```python
from build123d import *

# Parameters (mm, degrees)
SKETCH2_W                      = 99
SKETCH2_H                      = 69
SKETCH2_R                      = 25
BOSS_EXTRUDE1_DEPTH            = 10
BOSS_EXTRUDE2_DEPTH            = 120
CBORE_FOR_M5_SHCS1_D           = 5.5
CBORE_FOR_M5_SHCS1_CBORE_D     = 8
CBORE_FOR_M5_SHCS1_CBORE_DEPTH = 7
M5_CLEARANCE_HOLE1_D           = 5.5
M5_CLEARANCE_HOLE2_D           = 5.5
M5_CLEARANCE_HOLE2_DEPTH       = 10
SKETCH11_W                     = 10
SKETCH11_H                     = 120
BOSS_EXTRUDE3_DEPTH            = 13.5
FILLET1_R                      = 20
FILLET2_R                      = 10


with BuildPart() as part:
    # Sketch2 → Boss-Extrude1 (new body)
    with BuildSketch(Plane(origin=(0, 0, 0), x_dir=(1, 0, 0), z_dir=(0, 1, 0))):
        with Locations((0, -4.5)):
            Rectangle(SKETCH2_W, SKETCH2_H)
        with Locations(Location((0, 0, 0), (0, 0, 270))):
            Circle(SKETCH2_R, mode=Mode.SUBTRACT)
    extrude(amount=BOSS_EXTRUDE1_DEPTH)

    # Sketch3 → Boss-Extrude2 (add)
    with BuildSketch(Plane.XZ):
        Polygon((-49.5, -30), (-49.5, 39), (49.5, 39), (49.5, -30), (39.5, -30), (39.5, 29), (-39.5, 29), (-39.5, -30), align=None)
    extrude(amount=BOSS_EXTRUDE2_DEPTH)

    # CBORE for M5 SHCS1 (through all)
    with Locations(Plane(origin=(0, 10, 0), x_dir=(1, 0, 0), z_dir=(0, 1, 0))):
        with Locations((24.748737342, 24.748737342), (-24.748737342, 24.748737342), (24.748737342, -24.748737342), (-24.748737342, -24.748737342)):
            CounterBoreHole(CBORE_FOR_M5_SHCS1_D / 2, CBORE_FOR_M5_SHCS1_CBORE_D / 2, CBORE_FOR_M5_SHCS1_CBORE_DEPTH)

    # M5 Clearance Hole1 (through all)
    with Locations(Plane.XY.offset(39)):
        with Locations((-12.5, -60), (12.5, -110), (-12.5, -110), (12.5, -60)):
            Hole(M5_CLEARANCE_HOLE1_D / 2)

    # M5 Clearance Hole2
    with Locations(Plane(origin=(49.5, 0, 0), x_dir=(0, 0, -1), z_dir=(1, 0, 0))):
        with Locations((0, -60), (0, -110)):
            Hole(M5_CLEARANCE_HOLE2_D / 2, depth=M5_CLEARANCE_HOLE2_DEPTH)

    # Sketch11 → Boss-Extrude3 (add)
    with BuildSketch(Plane(origin=(-39.5, 0, 0), x_dir=(0, 0, -1), z_dir=(1, 0, 0))):
        with Locations((25, -60)):
            Rectangle(SKETCH11_W, SKETCH11_H)
    extrude(amount=BOSS_EXTRUDE3_DEPTH)

    # Fillet1
    fillet1_edges = [part.edges().sort_by_distance(p)[0] for p in [
        (49.5, -55, 39),
        (-49.5, -55, 39),
    ]]
    fillet(fillet1_edges, radius=FILLET1_R)

    # Fillet2
    # the kernel refuses this fillet: 10 mm, written as the material it adds along each edge
    with BuildSketch(Plane(origin=(39.5, 0, -30), x_dir=(0, -1, 0), z_dir=(0, 0, 1))) as fillet2_piece_1:
        with BuildLine():
            CenterArc((FILLET2_R, -FILLET2_R), FILLET2_R, 90, 90)
            Line((0, -FILLET2_R), (0, 0))
            Line((0, 0), (FILLET2_R, 0))
        make_face()
    extrude(amount=59)
    with BuildSketch(Plane(origin=(-39.5, 0, 29), x_dir=(1, 0, 0), z_dir=(0, 0, -1))) as fillet2_piece_2:
        with BuildLine():
            CenterArc((FILLET2_R, FILLET2_R), FILLET2_R, 180, 90)
            Line((0, FILLET2_R), (0, 0))
            Line((0, 0), (FILLET2_R, 0))
        make_face()
    extrude(amount=49)
    with BuildSketch(Plane(origin=(-39.5, 0, 29), x_dir=(0, 0, -1), z_dir=(0, -1, 0))) as fillet2_piece_3:
        with BuildLine():
            CenterArc((FILLET2_R, FILLET2_R), FILLET2_R, 180, 90)
            Line((0, FILLET2_R), (0, 0))
            Line((0, 0), (FILLET2_R, 0))
        make_face()
    extrude(amount=120)
    with BuildSketch(Plane(origin=(39.5, 0, 29), x_dir=(0, 0, -1), z_dir=(0, -1, 0)), Plane(origin=(-39.5, -120, -20), x_dir=(1, 0, 0), z_dir=(0, 1, 0))) as fillet2_piece_4:
        with BuildLine():
            CenterArc((FILLET2_R, -FILLET2_R), FILLET2_R, 90, 90)
            Line((0, -FILLET2_R), (0, 0))
            Line((0, 0), (FILLET2_R, 0))
        make_face()
    extrude(amount=120)
    with BuildSketch(Plane(origin=(-26, 0, -2.197582327), x_dir=(1, 0, 0), z_dir=(0, 0, -1))) as fillet2_piece_5_section:
        with BuildLine():
            CenterArc((FILLET2_R, FILLET2_R), FILLET2_R, 180, 90)
            Line((0, FILLET2_R), (0, 0))
            Line((0, 0), (FILLET2_R, 0))
        make_face()
    fillet2_piece_5 = extrude(amount=27.802417673, mode=Mode.PRIVATE)
    fillet2_piece_5 = split(fillet2_piece_5, bisect_by=Plane(origin=(-18.601224516, -0.292097945, -20), z_dir=(0, 0, -1)), keep=Keep.TOP, mode=Mode.PRIVATE)
    fillet2_piece_5 = fillet2_piece_5 - Plane(origin=(-24.748737342, -0.292097945, -24.748737342), x_dir=(-1, 0, 0), z_dir=(0, -1, 0)) * Cylinder(2.75, 96, mode=Mode.PRIVATE)
    add(fillet2_piece_5)


solid = part.part
```
Input: part model. Units: mm. Frame: model coordinates. A direction names the side the tool comes from. Coordinates: 2 decimals unless noted, no trailing zeros. Order: outer loops, then holes, each group sorted by start corner. A loop starts at its lowest first (then second) coordinate and runs counter-clockwise, first axis right, second up. Notation, with made-up numbers: (-13.5, 35) - (12.5, 35) arc R16 cw to (12.5, 64) - close; hole circle Ø9 at (44.25, 65.5). An arc over 180 degrees is marked (long way). Put each result on its own line as item: value.
1. Cut plane B-B on z = 0. Return the cut outline in (x, y).
Report:
outline: (-49.5, -120) - (-39.5, -120) - (-39.5, -10) arc R10 cw to (-29.5, 0) - (-25, 0) - (-25, 10) - (-49.5, 10) - close; (25, 0) - (29.5, 0) arc R10 cw to (39.5, -10) - (39.5, -57.25) - (49.5, -57.25) - (49.5, 10) - (25, 10) - close; (39.5, -120) - (49.5, -120) - (49.5, -112.75) - (39.5, -112.75) - close; (39.5, -107.25) - (49.5, -107.25) - (49.5, -62.75) - (39.5, -62.75) - close
2. Cut plane D-D on z = 17.5. Return the cut outline in (x, y).
Report:
outline: (-49.5, -120) - (-39.5, -120) - (-39.5, -10) arc R10 cw to (-29.5, 0) - (-17.85, 0) - (-17.85, 10) - (-49.5, 10) - close; (17.85, 0) - (29.5, 0) arc R10 cw to (39.5, -10) - (39.5, -120) - (49.5, -120) - (49.5, 10) - (17.85, 10) - close
3. Line query: line 1 along Y through (x, z) = (-12.5, 35); line 2 along X through (y, z) = (-22, -24.5); line 3 along Y through (x, z) = (27, -1). Output: solid intervals per line, ascending.
Report:
line 1: y = -120 to -112.75, -107.25 to -62.75, -57.25 to 10
line 2: x = -49.5 to -26, 39.5 to 49.5
line 3: y = 0 to 10
4. Cut plane A-A on y = -60. Return the cut outline in (x, z), then the cut area to 3 significant figures.
Report:
outline: (-49.5, -30) - (-26, -30) - (-26, -20) - (-29.5, -20) arc R10 cw to (-39.5, -10) - (-39.5, 19) arc R10 cw to (-29.5, 29) - (-15.25, 29) - (-15.25, 39) - (-29.5, 39) arc R20 ccw to (-49.5, 19) - close; (-9.75, 29) - (9.75, 29) - (9.75, 39) - (-9.75, 39) - close; (15.25, 29) - (29.5, 29) arc R10 cw to (39.5, 19) - (39.5, 2.75) - (49.5, 2.75) - (49.5, 19) arc R20 ccw to (29.5, 39) - (15.25, 39) - close; (39.5, -30) - (49.5, -30) - (49.5, -2.75) - (39.5, -2.75) - close
area: 2,030 mm2
5. Draft query along Y for faces 1 (the face through (-12.142, -57.273, 33.93)), 2 (the face through (-22, 3, -26)), 3 (the face through (43.797, -54.09, 32.986)). Return one class per face: pulls with the +Y half, pulls with the -Y half, needs draft (parallel to the pull), parting line crosses it, or undercut.
Report:
face 1: undercut
face 2: pulls with the +Y half
face 3: needs draft
6. Reachability of faces 4 (the face through (-21.825, -1.872, -24.93)), 5 (the face through (28.564, 6.549, 23.547)), 6 (the face through (49.5, -54, -5)) from +Z, -Z, +X, -X, +Y, -Y: full face, straight path, thin tool, end or side. Return the list, or none.
Report:
face 4: -Z, -Y
face 5: +Y
face 6: +Z, -Z, +X, +Y, -Y
7. Contact query for flat-ended pins moving along their axis: pin 1 Ø1.2 at (x, z) = (-26.5, -25) entering from +Y; pin 2 Ø4 at (x, z) = (-25.5, -25.5) entering from +Y; pin 3 Ø3 at (x, z) = (-38.5, -1.5) entering from -Y; pin 4 Ø9 at (x, y) = (-12.5, -110) entering from -Z. Output: stop coordinate, or through.
Report:
pin 1: stops at y = 0
pin 2: stops at y = 3
pin 3: stops at y = -120
pin 4: stops at z = 29
8. Cut plane C-C on x = 0. Return the cut outline in (y, z).
Report:
outline: (-120, 29) - (0, 29) - (0, 25) - (10, 25) - (10, 39) - (-120, 39) - close; (0, -30) - (10, -30) - (10, -25) - (0, -25) - close
